Can you work these out from the model? Positions are in its coordinate system, mm. Round coordinates to 2 decimals unless told otherwise and drop trailing zeros. Answer as a JSON object with one key per item and string values.
Autodesk Inventor part; units mm, degrees
ref_plane "Work Plane1" through (0, 0, -66) normal (0, 0, -1) x (-1, 0, 0)
ref_plane "YZ Plane" through (0, 0, 0) normal (1, 0, 0) x (0, 1, 0)
ref_plane "XZ Plane" through (0, 0, 0) normal (0, 1, 0) x (-1, 0, 0)
sketch "Sketch1" plane through (0, 0, 0) normal (0, 0, 1) x (1, 0, 0)
  line L0 (-236.5, -142.5) -> (236.5, -142.5)
  line L1 (236.5, -142.5) -> (236.5, 142.5)
  line L2 (236.5, 142.5) -> (-236.5, 142.5)
  line L3 (-236.5, 142.5) -> (-236.5, -142.5)
  line L4 (-236.5, -142.5) -> (236.5, 142.5) construction
  line L5 (236.5, -142.5) -> (-236.5, 142.5) construction
  point P0 (0, 0)
  dimension "d0" = 473
  dimension "d1" = 285
extrude "Extrusion1" add sketch "Sketch1" against normal blind 26
sketch "Sketch2" plane through (0, 0, -26) normal (0, 0, -1) x (-1, 0, 0)
  line L0 (-233.5, -139.5) -> (233.5, -139.5)
  line L1 (233.5, -139.5) -> (233.5, 139.5)
  line L2 (233.5, 139.5) -> (-233.5, 139.5)
  line L3 (-233.5, 139.5) -> (-233.5, -139.5)
  line L4 (-233.5, -139.5) -> (233.5, 139.5) construction
  line L5 (233.5, -139.5) -> (-233.5, 139.5) construction
  line L6 (236.5, 142.5) -> (-236.5, 142.5)
  line L7 (-236.5, 142.5) -> (-236.5, -142.5)
  point P0 (0, 0)
  dimension "d4" = 3
  dimension "d5" = 3
ref_plane "Work Plane1" through (0, 0, -66) normal (0, 0, -1) x (-1, 0, 0)
sketch "Sketch4" plane through (0, 0, -66) normal (0, 0, -1) x (-1, 0, 0)
  line L0 (-190, -70) -> (190, -70)
  line L1 (190, -70) -> (190, 70)
  line L2 (190, 70) -> (-190, 70)
  line L3 (-190, 70) -> (-190, -70)
  line L4 (-190, -70) -> (190, 70) construction
  line L5 (190, -70) -> (-190, 70) construction
  point P0 (0, 0)
  dimension "d7" = 140
  dimension "d8" = 380
loft "Loft1" add profiles "Sketch2", "Sketch4"
sketch "Sketch5" plane through (190, -70, -66) normal (0, 0, -1) x (-1, 0, 0)
  line L0 (140, 20) -> (240, 20)
  line L1 (240, 20) -> (240, 120)
  line L2 (240, 120) -> (140, 120)
  line L3 (140, 120) -> (140, 20)
  line L4 (140, 20) -> (240, 120) construction
  line L5 (240, 20) -> (140, 120) construction
  point P0 (190, 70)
  dimension "d13" = 100
  dimension "d14" = 100
hole "Hole1" at (50, 50, -66) at (-50, 50, -66) at (-50, -50, -66) at (50, -50, -66) direction (0, 0, 1) diameter 4.134 depth 15 tip angle 118
sketch "Sketch6" plane through (0, 0, 0) normal (0, 0, 1) x (1, 0, 0)
  line L0 (-221.5, -127.5) -> (221.5, -127.5)
  line L1 (221.5, -127.5) -> (221.5, 127.5)
  line L2 (221.5, 127.5) -> (-221.5, 127.5)
  line L3 (-221.5, 127.5) -> (-221.5, -127.5)
  line L4 (-221.5, -127.5) -> (221.5, 127.5) construction
  line L5 (221.5, -127.5) -> (-221.5, 127.5) construction
  line L6 (236.5, 142.5) -> (-236.5, 142.5)
  line L7 (-236.5, 142.5) -> (-236.5, -142.5)
  point P0 (0, 0)
  dimension "d22" = 15
  dimension "d23" = 15
extrude "Extrusion2" cut sketch "Sketch6" against normal blind 4
properties part number "Monitor_21inch"
Q1. If I drill on L1, parallel to X at y = 50, z = -58; L2, parallel to X at y = -50, z = -63; L3, parallel to Y at x = 50, z = -58.25, over which ranges is the centre line in solid material (lowest first)? Write a range as [from, to].
Determined:
{"L1": "[-198.7, -52.07], [-47.93, 47.93], [52.07, 198.7]", "L2": "[-193.26, -52.07], [-47.93, 47.93], [52.07, 193.26]", "L3": "[-83.47, -52.07], [-47.93, 47.93], [52.07, 83.47]"}
Q2. I'm going to push flat-ended pins straight in: pin 1 (5 mm diameter, centred on x = -11, z = -50, fed in from -Y); pin 2 (2 mm diameter, centred on x = 98, z = -41.5, fed in from -Y); pin 3 (8 mm diameter, centred on x = -49, z = -30.5, fed in from +Y). Where does each tip first touch, or does it pass through?
Determined:
{"pin 1": "y = -102.14", "pin 2": "y = -114.31", "pin 3": "y = 138.63"}
Q3. We'd pull the mould along X, two halves only. Please class faces 1 (the flat face through (-19, -137, 0)), 2 (the flat face through (-3, 2, -4)), 3 (the flat face through (-236.5, 2, -13)), 4 (the flat face through (236.5, -2, -13)): pulls with the +X half, pulls with the -X half, needs draft (parallel to the pull), parting line crosses it, or undercut.
Determined:
{"face 1": "needs draft", "face 2": "undercut", "face 3": "pulls with the -X half", "face 4": "pulls with the +X half"}
